Check sheet for the modelled part. Datum: model origin and axes. Units: mm. Coordinates: 2 decimals unless noted, no trailing zeros. Loops run counter-clockwise (first coordinate to the right, second up) from the corner with the lowest first, then second, coordinate; pieces in that order, holes last. Notation, with made-up numbers: (-22.75, 18.25) - (-4.75, 18.25) arc R34 cw to (-4.75, 48.25) - close; hole circle Ø6 at (-39.75, 21.25). An arc over 180 degrees is marked (long way). Answer as a JSON object with one key per item and string values. Group by question number.
from build123d import *

# Parameters (mm, degrees)
F1_DEPTH     = 75
F2_T         = -6
F3_W         = 75
F3_H         = 75
F4_DEPTH     = 1000
F6_W         = 75
F6_H         = 75
F7_DEPTH     = 1000
F9_DEPTH     = 75
F11_DEPTH    = 75
F12_T        = 6
F12_T3_DEPTH = 87
F12_T6_ANGLE = 180.000000001
F12_T8_ANGLE = 180.000000001


# Not quite as in the source:
# - a shell that OpenCascade refuses in one call is made with other operations: the cavity is built on its own and cut out


with BuildPart() as f1:
    # F0 (on Front) → F1 (new body)
    with BuildSketch(Plane.XZ):
        with BuildLine():
            ThreePointArc((707.1067811865, 707.1067811865), (923.8795325113, 382.6834323651), (1000, 0))
            Line((1000, 0), (1050, 0))
            ThreePointArc((1050, 0), (0, 1050), (-1050, 0))
            Line((-1050, 0), (-1000, 0))
            ThreePointArc((-1000, 0), (-923.8795325113, 382.6834323651), (-707.1067811865, 707.1067811865))
            ThreePointArc((-707.1067811865, 707.1067811865), (-382.6834323651, 923.8795325113), (0, 1000))
            ThreePointArc((0, 1000), (382.6834323651, 923.8795325113), (707.1067811865, 707.1067811865))
        make_face()
    extrude(amount=F1_DEPTH)

    # F2
    f2_openings = [f1.faces().sort_by_distance(p)[0] for p in [
        (0, -37.5, 1050),
        (1025, -37.5, 0),
        (-1025, -37.5, 0),
    ]]
    offset(amount=F2_T, openings=f2_openings)

    # F3 (on Right) → F4 (join)
    with BuildSketch(Plane.YZ):
        with Locations((-37.5, 37.5)):
            Rectangle(F3_W, F3_H)
    extrude(amount=F4_DEPTH)

    # F5: F1 across plane


with BuildPart() as f1_1:
    add(f1.part)
    add(f1.part.mirror(Plane.YZ))

    # F6 (on face) → F7 (join)
    with BuildSketch(Plane(origin=(0, 0, 0), x_dir=(1, 0, 0), z_dir=(0, 0, -1))):
        with Locations((0, 37.5)):
            Rectangle(F6_W, F6_H)
    extrude(amount=-F7_DEPTH)

    # F8 (on face) → F9 (join)
    with BuildSketch(Plane.XZ):
        with BuildLine():
            Line((84.9014701911, 30.3333466038), (733.1259261111, 680.0929175221))
            ThreePointArc((733.1259261111, 680.0929175221), (707.1120975666, 707.1120975666), (680.0929175221, 733.1259261111))
            Line((680.0929175221, 733.1259261111), (-22.6996619852, 30.3333466038))
            Line((-22.6996619852, 30.3333466038), (84.9014701911, 30.3333466038))
        make_face()
        Polygon((-27.0138636644, 26.0191449246), (-22.6996619852, 30.3333466038), (-27.0138636644, 30.3333466038), align=None)
    extrude(amount=F9_DEPTH)

    # F10 (on Front) → F11 (join)
    with BuildSketch(Plane.XZ):
        Polygon((-97.2271824132, 44.1941738242), (-27.4779913529, 44.1941738242), (-30.0520382004, 83.0850467894), (-680.5902768921, 733.623285481), (-733.623285481, 680.5902768921), align=None)
    extrude(amount=F11_DEPTH)

    # F12: shell of thickness 6, made by hand


with BuildPart() as f12_core1:
    # F12_t2: copy of F1
    add(f1_1.part)

    # the walls: a layer under each face that stays
    f12_faces = [f12_core1.faces().sort_by_distance(p)[0] for p in [
        (0, 0, 525),
        (0, -37.5, 0),
        (0, -3, 1050),
        (-562.608271174, -37.5, 75),
        (-37.5, -37.5, 544.9148181113),
        (-382.6834323651, -37.5, 923.8795325113),
        (-916.5299048246, -37.5, 399.9661655218),
        (563.3230641949, -37.5, 75),
        (431.2942603709, -37.5, 377.5464587611),
        (916.5299048246, -37.5, 399.9661655218),
        (382.6834323651, -37.5, 923.8795325113),
        (37.5, -37.5, 544.9148181113),
        (358.7964587611, -37.5, 411.82946735),
        (-900, -6, 525),
        (0, -37.5, 1006),
        (-900, -69, 525),
        (0, -72, 1050),
        (0, -75, 525),
        (-430.57946735, -37.5, 377.5464587611),
        (-358.7964587611, -37.5, 411.82946735),
    ]]
    thicken(f12_faces, amount=-F12_T, mode=Mode.SUBTRACT)

    # F12_s4 → F12_t3 (cut)
    with BuildSketch(Plane.XZ.offset(-6)):
        Polygon((-128.0754349959, 75.0175735931), (-128.033008589, 69), (-113.5477272148, 69), (-123.7903679019, 79.2426406871), align=None)
        Polygon((-997.1237027469, 75.0555), (-997.183533759, 69), (-1003.6517512752, 69), (-1003.1666349615, 75.45), align=None)
        Polygon((-37.5175735931, 90.5754349959), (-31.5, 90.533008589), (-31.5, 76.0477272148), (-41.7426406871, 86.2903679019), align=None)
        Polygon((-37.55775, 999.236669836), (-31.5, 999.2966276337), (-31.5, 1005.5260092085), (-37.725, 1005.2924073995), align=None)
        Polygon((-680.0096855402, 733.1243649624), (-684.1734750272, 737.5246816678), (-688.7403961634, 733.2881233782), (-684.3355582092, 728.883285424), align=None)
        Polygon((-733.1243649624, 680.0096855402), (-737.5246816678, 684.1734750272), (-733.2881233782, 688.7403961634), (-728.883285424, 684.3355582092), align=None)
        Polygon((997.1237027469, 75.0555), (997.183533759, 69), (1003.6517512752, 69), (1003.1666349615, 75.45), align=None)
        Polygon((129.5050711853, 75.0176238001), (129.4625946308, 69), (115.0015064822, 69), (125.2149391782, 79.2376199873), align=None)
        Polygon((733.1244151101, 680.0097357472), (728.8782706586, 684.3305375094), (733.2831062303, 688.7458045437), (737.5246816678, 684.1734750272), align=None)
        Polygon((680.0096855402, 733.1243649624), (684.1734750272, 737.5246816678), (688.7403961634, 733.2881233782), (684.3355582092, 728.883285424), align=None)
        Polygon((37.55775, 999.236669836), (37.725, 1005.2924073995), (31.5, 1005.5260092085), (31.5, 999.2966276337), align=None)
        Polygon((37.5175735931, 90.5754349959), (31.5, 90.533008589), (31.5, 76.0477272148), (41.7426406871, 86.2903679019), align=None)
    extrude(amount=F12_T3_DEPTH, mode=Mode.SUBTRACT)

    # F12_s5 → F12_t6 (revolve, cut)
    with BuildSketch(Plane.XY):
        Polygon((-1006.06, -6.06), (-1006, 0), (-1000, 0), (-1000, -6), align=None)
    revolve(axis=Axis((0, -6, 0), (0, 1, 0)), revolution_arc=F12_T6_ANGLE, mode=Mode.SUBTRACT)

    # F12_s7 → F12_t8 (revolve, cut)
    with BuildSketch(Plane.XY):
        Polygon((-1006.06, -68.94), (-1000, -69), (-1000, -75), (-1006, -75), align=None)
    revolve(axis=Axis((0, -69, 0), (0, 1, 0)), revolution_arc=F12_T8_ANGLE, mode=Mode.SUBTRACT)


with BuildPart() as f1_2:
    add(f1_1.part)

    # what is left inside the walls is the cavity
    f12_cavity = [f12_core1.part.solids().sort_by_distance(p)[0] for p in [
        (0, -6.06, 337.333333),
    ]]
    add(f12_cavity, mode=Mode.SUBTRACT)


solid = f1_2.part
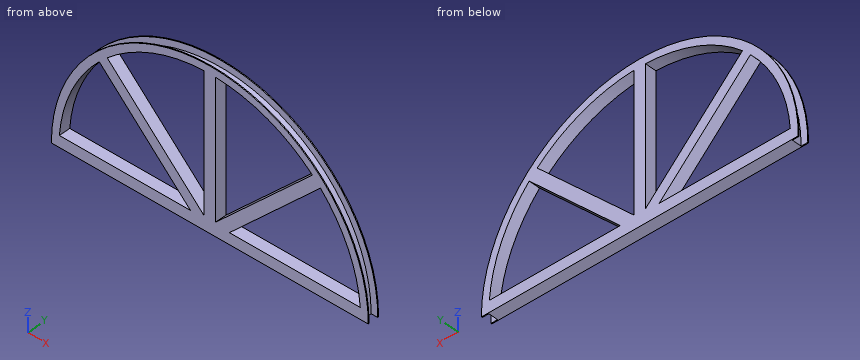
1. Sectioned sample at D-D on x = -759. Record the cut outline in (y, z), plus the area to 3 significant figures.
2. Sectioned sample at A-A on z = 809.5. Record the cut outline in (x, y).
3. Gauge pin test, flat ends, axial feed: pin 1 (4 mm diameter, centred on x = -456, y = -26.5, fed in from +Z); pin 2 (6 mm diameter, centred on y = -50, z = 872, fed in from -X); pin 3 (8 mm diameter, centred on y = -35, z = 364, fed in from +X). Record the tip position at first contact, or that the pin passes through.
4. Material ranges on line 1 (Z direction, x = -551.5, y = -28); line 2 (Z direction, x = -787, y = -21.5); line 3 (Z direction, x = 848.5, y = -17), recorded low to high.
5. Sectioned sample at B-B on x = 612.5. Record the cut outline in (y, z), plus the area to 3 significant figures.
6. Sectioned sample at C-C on y = -38.5. Record the cut outline in (x, z).
Answers follow:
{
 "1": {"outline": "(-75, 0) - (0, 0) - (0, 75) - (-75, 75) - close; (-75, 651.09) - (0, 651.09) - (0, 725.55) - (-6, 725.55) - (-6, 660.27) - (-69, 660.27) - (-69, 725.55) - (-75, 725.55) - close; hole (-69, 6) - (-6, 6) - (-6, 69) - (-69, 69) - close", "area": "3,130 mm^2"},
 "2": {"outline": "(-668.74, -75) - (-587.12, -75) - (-587.12, 0) - (-668.74, 0) - (-668.74, -6) - (-597.28, -6) - (-597.28, -69) - (-668.74, -69) - close; (-37.5, -75) - (37.5, -75) - (37.5, 0) - (-37.5, 0) - close; (587.12, -75) - (668.74, -75) - (668.74, -69) - (597.28, -69) - (597.28, -6) - (668.74, -6) - (668.74, 0) - (587.12, 0) - close; hole (-31.5, -69) - (31.5, -69) - (31.5, -6) - (-31.5, -6) - close"},
 "3": {"pin 1": "stops at z = 897.73", "pin 2": "stops at x = -506.83", "pin 3": "stops at x = 939.38"},
 "4": {"line 1": "z = 0 to 6, 69 to 75, 498.47 to 506.95, 596.05 to 604.53, 834.17 to 841.36", "line 2": "z = 0 to 6, 69 to 75, 616.95 to 626.63", "line 3": "z = 0 to 6, 69 to 75, 529.2 to 540.45"},
 "5": {"outline": "(-75, 0) - (0, 0) - (0, 75) - (-75, 75) - close; (-75, 559.18) - (0, 559.18) - (0, 665.53) - (-75, 665.53) - close; (-75, 790.47) - (0, 790.47) - (0, 852.84) - (-6, 852.84) - (-6, 798.05) - (-69, 798.05) - (-69, 852.84) - (-75, 852.84) - close; hole (-69, 6) - (-6, 6) - (-6, 69) - (-69, 69) - close; hole (-69, 567.68) - (-6, 567.68) - (-6, 657.05) - (-69, 657.05) - close", "area": "5,230 mm^2"},
 "6": {"outline": "(-1006, 0) - (1006, 0) arc R1006 ccw to start; hole (-999.98, 6) - (999.98, 6) arc R1000 ccw to (997.62, 69) - (115, 69) - (729.03, 684.48) arc R1000 ccw to (684.48, 729.03) - (31.5, 76.05) - (31.5, 999.5) arc R1000 ccw to (-31.5, 999.5) - (-31.5, 76.05) - (-684.48, 729.03) arc R1000 ccw to (-729.03, 684.48) - (-113.55, 69) - (-997.62, 69) arc R1000 ccw to start; hole (-997.18, 75) - (-128.03, 75) - (-733.13, 680.09) arc R1000 ccw to start; hole (-680.09, 733.13) - (-37.5, 90.53) - (-37.5, 999.3) arc R1000 ccw to start; hole (37.5, 90.53) - (680.09, 733.13) arc R1000 ccw to (37.5, 999.3) - close; hole (129.46, 75) - (997.18, 75) arc R1000 ccw to (733.13, 680.09) - close"}
}
